Input: part model. Units: mm. Frame: model coordinates. A direction names the side the tool comes from. Give positions to 0.01 mm unless a question says otherwise; leave off trailing zeros. Loops run counter-clockwise (first coordinate to the right, second up) from the corner with the lowest first, then second, coordinate; pieces in that order, holes last. Notation, with made-up numbers: M 7.5,10.25 L 54.5,10.25 A22 ccw 54.5,46.25 Z; hole C 66,85 d3. An arc over 180 degrees is marked long. Use a Markdown table: item, result. Add a question column.
from build123d import *

# Parameters (mm, degrees)
SKETCH1_R           = 7
BOSS_EXTRUDE1_DEPTH = 13
SHELL2_T            = -1
SKETCH2_R           = 2.5
CUT_EXTRUDE1_DEPTH  = 10
SKETCH3_R           = 9
BOSS_EXTRUDE2_DEPTH = 1
CUT_EXTRUDE2_START  = -2
SKETCH4_R           = 6
CUT_EXTRUDE2_DEPTH  = 2


with BuildPart() as part:
    # Sketch1 → Boss-Extrude1 (new body)
    with BuildSketch(Plane(origin=(0, 0, 0), x_dir=(1, 0, 0), z_dir=(0, 1, 0))):
        with Locations(Location((0, 0, 0), (0, 0, 90))):
            Circle(SKETCH1_R)
    extrude(amount=BOSS_EXTRUDE1_DEPTH)

    # Shell2
    shell2_openings = [part.faces().sort_by_distance(p)[0] for p in [
        (0, 13, 0),
    ]]
    offset(amount=SHELL2_T, openings=shell2_openings, kind=Kind.INTERSECTION)

    # Sketch2 → Cut-Extrude1 (cut)
    with BuildSketch(Plane.XZ):
        with Locations(Location((0, 0, 0), (0, 0, 270))):
            Circle(SKETCH2_R)
    extrude(amount=-CUT_EXTRUDE1_DEPTH, mode=Mode.SUBTRACT)

    # Sketch3 → Boss-Extrude2 (add)
    with BuildSketch(Plane(origin=(0, 13, 0), x_dir=(1, 0, 0), z_dir=(0, 1, 0))):
        with Locations(Location((0, 0, 0), (0, 0, 270))):
            Circle(SKETCH3_R)
    extrude(amount=BOSS_EXTRUDE2_DEPTH)

    # Sketch4 → Cut-Extrude2 (cut)
    with BuildSketch(Plane(origin=(0, 14, 0), x_dir=(1, 0, 0), z_dir=(0, 1, 0)).offset(CUT_EXTRUDE2_START)):
        with Locations(Location((0, 0, 0), (0, 0, 90))):
            Circle(SKETCH4_R)
    extrude(amount=CUT_EXTRUDE2_DEPTH, mode=Mode.SUBTRACT)


solid = part.part
1) Section query C-C, the plane y = 9.25. Return the cut outline in (x, z), and give its area (3 significant figures).
2) Reachability of faces 1 (the flat face through (-6, 14, 2)), 2 (the flat face through (0, 1, -3)) from +Z, -Z, +X, -X, +Y, -Y: full face, straight path, thin tool, end or side. Return the list, or none.
3) Pull-direction query (X, two-part tool) for faces 3 (the cylindrical face through (6.834, 6.409, 1.517)), 4 (the flat face through (-7.3, 13, 0)), 5 (the cylindrical face through (-1.802, 7.409, -5.723)); classes: pulls with the +X half, pulls with the -X half, needs draft (parallel to the pull), parting line crosses it, or undercut.
4) Section query A-A, the plane x = 0. Return the cut outline in (y, z).
5) Ray query, line 1 (X direction, y = 0.3, z = 0); line 2 (X direction, y = 2.25, z = 0); line 3 (Y direction, x = -1.75, z = 5.5). Return the intervals inside material, ascending. Write a range as [from, to].
6) Section query B-B, the plane z = 0. Return the cut outline in (x, y).
7) Section query D-D, the plane z = 3.5. Return the cut outline in (x, y).
8) Contact query for flat-ended pins moving along their axis: P1, Ø4, axis at x = 5.5, y = 5, coming from the -Z side; P2, Ø3.5, axis at x = -1.5, z = 1.5, coming from the +Y side; P3, Ø5, axis at x = 5, y = 9, coming from the +Z side. Output: stop coordinate, or through.
Entries:
| question | item | result |
|---|---|---|
| 1 | outline | C 0,0 d14; hole C 0,0 d12 |
| 1 | area | 40.8 mm² |
| 2 | face 1 | +Z, -Z, +X, -X, +Y |
| 2 | face 2 | +Y |
| 3 | face 3 | parting line crosses it |
| 3 | face 4 | needs draft |
| 3 | face 5 | undercut |
| 4 | outline | M 0,-7 L 13,-7 L 13,-9 L 14,-9 L 14,-6 L 1,-6 L 1,-2.5 L 0,-2.5 Z; M 0,2.5 L 1,2.5 L 1,6 L 14,6 L 14,9 L 13,9 L 13,7 L 0,7 Z |
| 5 | line 1 | x = [-7, -2.5], [2.5, 7] |
| 5 | line 2 | x = [-7, -6], [6, 7] |
| 5 | line 3 | y = [0, 1] |
| 6 | outline | M -9,13 L -7,13 L -7,0 L -2.5,0 L -2.5,1 L -6,1 L -6,14 L -9,14 Z; M 2.5,0 L 7,0 L 7,13 L 9,13 L 9,14 L 6,14 L 6,1 L 2.5,1 Z |
| 7 | outline | M -8.29,13 L -6.06,13 L -6.06,0 L 6.06,0 L 6.06,13 L 8.29,13 L 8.29,14 L 4.87,14 L 4.87,1 L -4.87,1 L -4.87,14 L -8.29,14 Z |
| 8 | P1 | stops at z = -6.06 |
| 8 | P2 | stops at y = 1 |
| 8 | P3 | stops at z = 6.54 |
